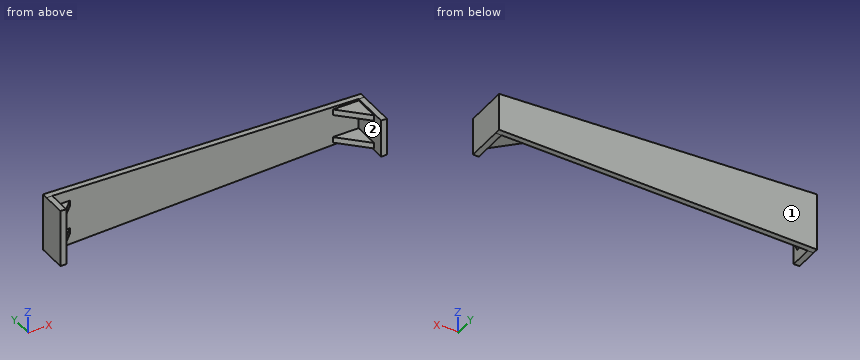
```python
from build123d import *

# Parameters (mm, degrees)
BOSS_EXTRUDE1_DEPTH     = 2
BOSS_EXTRUDE2_DEPTH     = 13
CUT_EXTRUDE1_DEPTH      = 58.879184514
CUT_EXTRUDE1_DEPTH_BACK = 58.879184514
BOSS_EXTRUDE3_START     = 4
BOSS_EXTRUDE3_DEPTH     = 2


with BuildPart() as part:
    # Sketch2 → Boss-Extrude1 (new body)
    with BuildSketch(Plane(origin=(0, 0, 0), x_dir=(1, 0, 0), z_dir=(0, 1, 0))):
        Polygon((55, -6.5), (-55, -10), (-55, 10), (55, 6.5), align=None)
    extrude(amount=-BOSS_EXTRUDE1_DEPTH)

    # Sketch3 → Boss-Extrude2 (add)
    with BuildSketch(Plane.XZ.offset(2)):
        Polygon((-53, 9.936363636), (-53, -9.936363636), (-55, -10), (-55, 10), align=None)
        Polygon((53, -6.563636364), (53, 6.563636364), (55, 6.5), (55, -6.5), align=None)
    extrude(amount=BOSS_EXTRUDE2_DEPTH)

    # Sketch5 → Cut-Extrude1 (cut, two sides: drawn at the far end of the back side and taken through both)
    with BuildSketch(Plane.XY.offset(-CUT_EXTRUDE1_DEPTH_BACK)):
        Polygon((-55, -10), (55, -15), (55, -25), (-55, -25), align=None)
    extrude(amount=CUT_EXTRUDE1_DEPTH + CUT_EXTRUDE1_DEPTH_BACK, mode=Mode.SUBTRACT)

    # Sketch6 → Boss-Extrude3 (add)
    with BuildSketch(Plane.XY.offset(BOSS_EXTRUDE3_START)):
        Polygon((-53, -8.090909091), (-46.909090909, -2), (-53, -2), align=None)
        Polygon((53, -10.909090909), (53, -2), (44.090909091, -2), align=None)
    boss_extrude3 = extrude(amount=BOSS_EXTRUDE3_DEPTH)

    # Mirror1: Boss-Extrude3 across plane
    add(boss_extrude3.mirror(Plane.XY))


solid = part.part
```
The model under review builds one solid part; all positions refer to its coordinate system, in mm. Face numbers are marked on the shaded views. Round coordinates to 2 decimals unless told otherwise and drop trailing zeros. Loops run counter-clockwise (first coordinate to the right, second up) from the corner with the lowest first, then second, coordinate; pieces in that order, holes last.
1) Clearance check with flat-ended pins moving along their axes: P1, Ø4, axis at x = 0, z = 4.5, coming from the +Y side; P2, Ø1.8, axis at x = -51, y = -5, coming from the -Z side; P3, Ø3, axis at x = -50.5, y = -6, coming from the +Z side; P4, Ø6, axis at x = -17, z = -3.5, coming from the -Y side. State where each tip first meets the part, or that it passes through.
Values follow:
P1: stops at y = 0
P2: stops at z = -6
P3: stops at z = 6
P4: stops at y = -2
2) Consider section A-A on z = -1. State the section outline as (x, y) points, then the cut area to 3 significant figures.
Values follow:
outline: (-55, -10) - (-53, -10.09) - (-53, -2) - (53, -2) - (53, -14.91) - (55, -15) - (55, 0) - (-55, 0) - close
area: 262 mm2
3) Consider section D-D on y = -4. State the section outline as (x, z) points, then the cut area to 3 significant figures.
Values follow:
outline: (-55, -10) - (-53, -9.94) - (-53, -6) - (-48.91, -6) - (-48.91, -4) - (-53, -4) - (-53, 4) - (-48.91, 4) - (-48.91, 6) - (-53, 6) - (-53, 9.94) - (-55, 10) - close; (46.09, -6) - (53, -6) - (53, -6.56) - (55, -6.5) - (55, 6.5) - (53, 6.56) - (53, 6) - (46.09, 6) - (46.09, 4) - (53, 4) - (53, -4) - (46.09, -4) - close
area: 110 mm2
4) Wall thickness on line 1 along X through (y, z) = (-4, -6.25); line 2 along Y through (x, z) = (-28.5, 0.25); line 3 along X through (y, z) = (-5.5, -8.25): over which ranges is each line inside the solid? List them lowest first.
Values follow:
line 1: x = -55 to -53, 53 to 55
line 2: y = -2 to 0
line 3: x = -55 to -53
5) Consider section B-B on y = -9. State the section outline as (x, z) points.
Values follow:
outline: (-55, -10) - (-53, -9.94) - (-53, 9.94) - (-55, 10) - close; (51.09, -6) - (53, -6) - (53, -6.56) - (55, -6.5) - (55, 6.5) - (53, 6.56) - (53, 6) - (51.09, 6) - (51.09, 4) - (53, 4) - (53, -4) - (51.09, -4) - close
6) Consider section C-C on x = 22. State the section outline as (y, z) points, then the cut area to 3 significant figures.
Values follow:
outline: (-2, -7.55) - (0, -7.55) - (0, 7.55) - (-2, 7.55) - close
area: 30.2 mm2
7) The part is to be moulded in two halves that separate along Z. For the marked faces 1 and 2, say which applies: pulls with the +Z half, pulls with the -Z half, needs draft (parallel to the pull), parting line crosses it, or undercut.
Values follow:
face 1: needs draft
face 2: undercut
